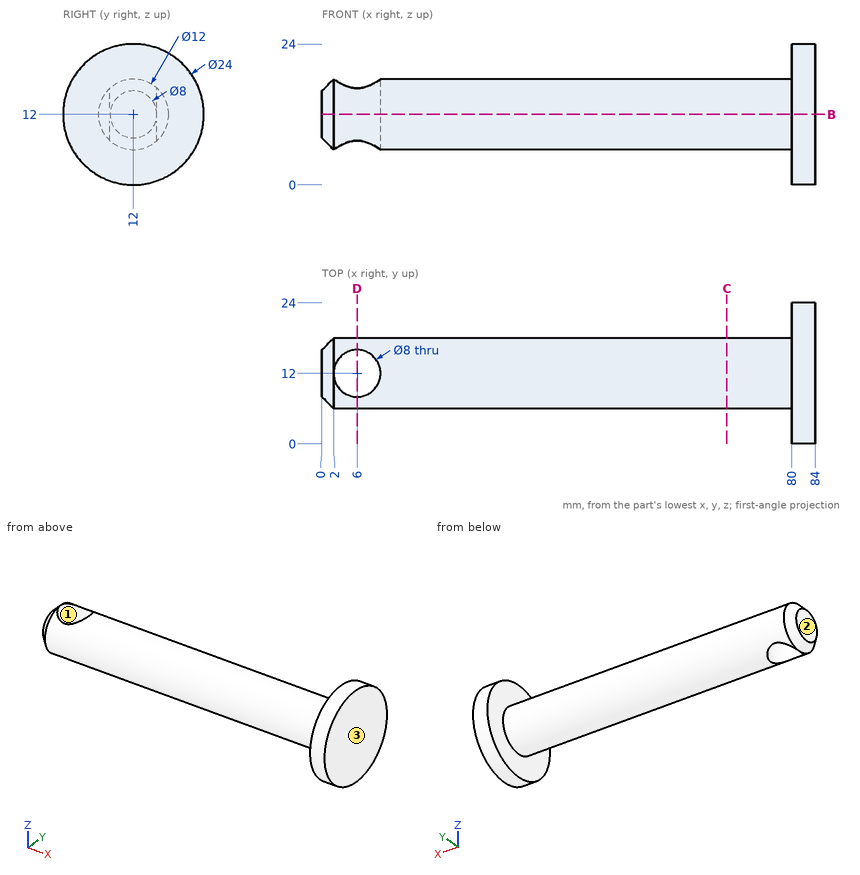
Design review of the part shown in the three views and the two pictorial views. Dimensions are in mm from the part's minimum x, y and z. Give positions to 0.01 mm unless a question says otherwise; leave off trailing zeros. Loops run counter-clockwise (first coordinate to the right, second up) from the corner with the lowest first, then second, coordinate; pieces in that order, holes last. Notation, with made-up numbers: M 74,0.25 L 123,0.25 A21 ccw 123,15.25 Z; hole C -12.5,13 d2. An arc over 180 degrees is marked long. Answer as a JSON object with one key per item and string values.
Item 1: Wall thickness on line 1 along X through (y, z) = (11.75, 8.25); line 2 along X through (y, z) = (11, 18.75); line 3 along Y through (x, z) = (6, 10.25): over which ranges is each line inside the solid? List them lowest first.
Output values:
{"line 1": "x = 0 to 2.01, 9.99 to 84", "line 2": "x = 80 to 84", "line 3": "y = 6.26 to 8, 16 to 17.74"}
Item 2: We need section B-B (z = 12). State the section outline as (x, y) points.
Output values:
{"outline": "M 0,8 L 2,6 L 80,6 L 80,0 L 84,0 L 84,24 L 80,24 L 80,18 L 2,18 L 0,16 Z; hole C 6,12 d8"}
Item 3: We need section D-D (x = 6). State the section outline as (y, z) points, and give its area (3 significant figures).
Output values:
{"outline": "M 8,7.53 L 8,16.47 A6 ccw Z; M 16,7.53 A6 ccw 16,16.47 Z", "area": "24.8 mm2"}
Item 4: We need section C-C (x = 69). State the section outline as (y, z) points, and give its area (3 significant figures).
Output values:
{"outline": "C 12,12 d12", "area": "113 mm2"}
Item 5: For P1, Ø5, axis at x = 55, z = 2.5, coming from the -Y side; P2, Ø12, axis at x = 41.5, y = 11.5, coming from the -Z side; P3, Ø1.5, axis at y = 13, z = 20.5, coming from the -X side; P4, Ø1, axis at x = 26, y = 6.5, coming from the +Z side, all flat-tipped, find the tip position at first contact; note any pin that passes through.
Output values:
{"P1": "passes through", "P2": "stops at z = 6", "P3": "stops at x = 80", "P4": "stops at z = 15.32"}
Item 6: Mouldability with a two-part tool opening along X and no side actions: class the marked faces 1, 2 and 3 as pulls with the +X half, pulls with the -X half, needs draft (parallel to the pull), parting line crosses it, or undercut.
Output values:
{"face 1": "undercut", "face 2": "pulls with the -X half", "face 3": "pulls with the +X half"}
